Here's how the part is built. I have some questions about the finished solid (model axes, mm). Coordinates: 2 decimals unless noted, no trailing zeros. Write each loop counter-clockwise with the first axis right and the second up, starting at its lowest first coordinate (ties: lowest second). Pieces come first, ordered by that corner, then holes.
Item 1: I want a section at A-A (y = 0). Please give me the cut outline in (x, z) (3 decimals), and give its area (3 significant figures).
Item 2: I want a section at B-B (x = 1.75). Please give me the cut outline in (y, z).
Item 3: If we mould it in two halves opening along Y, with no side actions, what happens to faces 1 (the face through (3.21, -5.04, 1.97)), 2 (the face through (0.56, -2.12, 1.97)), 3 (the face through (1.2, -1.2, 4))? For each: pulls with the +Y half, pulls with the -Y half, needs draft (parallel to the pull), parting line crosses it, or undercut.
Item 4: I'm going to push flat-ended pins straight in: P1, Ø5, axis at x = -1.5, y = 2, coming from the -Z side; P2, Ø2.5, axis at x = 1.75, y = -3.03, coming from the +Z side (1 decimal). Where does each tip first touch, or does it pass through?
Item 5: I want a section at C-C (x = 0). Please give me the cut outline in (y, z) (3 decimals).
Item 6: I want a section at D-D (y = 3.5). Please give me the cut outline in (x, z), and give its area (3 significant figures).
Item 7: Please list where these lines run through material, in increasing order: line 1 (Y direction, x = 2.75, z = 0.3); line 2 (X direction, y = 0.75, z = 1.45); line 3 (Y direction, x = 2, z = 3.25).
Autodesk Inventor part; units mm, degrees
ref_plane "YZ Plane" through (0, 0, 0) normal (1, 0, 0) x (0, 1, 0)
ref_plane "XZ Plane" through (0, 0, 0) normal (0, 1, 0) x (-1, 0, 0)
ref_plane "XY Plane" through (0, 0, 0) normal (0, 0, 1) x (1, 0, 0)
sketch "スケッチ1" plane through (0, 0, 0) normal (0, 0, 1) x (1, 0, 0)
  circle A0 centre (0, 0) radius 1.5
  circle A1 centre (1.75, 3.0311) radius 1.5
  circle A2 centre (-3.5, 0) radius 1.5
  circle A3 centre (1.75, -3.0311) radius 1.5
  circle A4 centre (0, 0) radius 5.975
  circle A5 centre (0, 0) radius 1.25 construction
  line L0 (-3.5, 0) -> (1.75, 3.0311) construction
  line L1 (1.75, 3.0311) -> (1.75, -3.0311) construction
  line L2 (1.75, -3.0311) -> (-3.5, 0) construction
  line L3 (0, 0) -> (3.1471, 0) construction
  circle A6 centre (0, 0) radius 3.5 construction
  dimension "d0" = 11.95
  dimension "d1" = 3
  dimension "d2" = 3
  dimension "d3" = 3.5
extrude "押し出し1" add sketch "スケッチ1" along normal blind 4
equation "\"d1\" = d2"
equation "\"d5\" = d6"
properties part number "原動節-ヘッケン接続部v2" material "アルミニウム 2014-T4"
Answer:
1. outline: (-5.975, 0) - (-5, 0) - (-5, 4) - (-5.975, 4) - close; (-2, 0) - (-1.5, 0) - (-1.5, 4) - (-2, 4) - close; (1.5, 0) - (5.975, 0) - (5.975, 4) - (1.5, 4) - close
1. area: 23.8 mm2
2. outline: (-5.71, 0) - (-4.53, 0) - (-4.53, 4) - (-5.71, 4) - close; (-1.53, 0) - (1.53, 0) - (1.53, 4) - (-1.53, 4) - close; (4.53, 0) - (5.71, 0) - (5.71, 4) - (4.53, 4) - close
3. face 1: parting line crosses it
3. face 2: undercut
3. face 3: needs draft
4. P1: stops at z = 0
4. P2: passes through
5. outline: (-5.975, 0) - (-1.5, 0) - (-1.5, 4) - (-5.975, 4) - close; (1.5, 0) - (5.975, 0) - (5.975, 4) - (1.5, 4) - close
6. outline: (-4.84, 0) - (0.33, 0) - (0.33, 4) - (-4.84, 4) - close; (3.17, 0) - (4.84, 0) - (4.84, 4) - (3.17, 4) - close
6. area: 27.3 mm2
7. line 1: y = -5.3 to -4.15, -1.91 to 1.91, 4.15 to 5.3
7. line 2: x = -5.93 to -4.8, -2.2 to -1.3, 1.3 to 5.93
7. line 3: y = -5.63 to -4.51, -1.55 to 1.55, 4.51 to 5.63
